Autodesk Inventor part; units mm, degrees
ref_plane "YZ Plane" through (0, 0, 0) normal (1, 0, 0) x (0, 1, 0)
ref_plane "XZ Plane" through (0, 0, 0) normal (0, 1, 0) x (-1, 0, 0)
ref_plane "XY Plane" through (0, 0, 0) normal (0, 0, 1) x (1, 0, 0)
sketch "Sketch1" plane through (0, 0, 0) normal (1, 0, 0) x (0, 1, 0)
  line L0 (0, 0) -> (57.15, 0)
  line L1 (57.15, 0) -> (57.15, 27.94)
  line L2 (0, 0) -> (0, 27.94)
  arc A0 (8.89, 27.94) -> (48.26, 27.94) centre (28.575, 49.4224) ccw
  line L3 (28.575, 0) -> (28.575, 8.5438) construction
  circle A1 centre (3.81, 3.81) radius 1.4
  circle A2 centre (53.34, 3.81) radius 1.4
  line L4 (0, 27.94) -> (5.08, 27.94)
  line L5 (5.08, 27.94) -> (5.08, 26.67)
  line L6 (5.08, 26.67) -> (7.62, 26.67)
  line L7 (7.62, 26.67) -> (7.62, 27.94)
  line L8 (7.62, 27.94) -> (8.89, 27.94)
  line L9 (57.15, 27.94) -> (52.07, 27.94)
  line L10 (52.07, 27.94) -> (52.07, 26.67)
  line L11 (52.07, 26.67) -> (49.53, 26.67)
  line L12 (49.53, 26.67) -> (49.53, 27.94)
  line L13 (49.53, 27.94) -> (48.26, 27.94)
  circle A3 centre (53.34, 24.13) radius 1.4
  circle A4 centre (3.81, 24.13) radius 1.4
  dimension "d0" = 57.15
  dimension "d1" = 27.94
  dimension "d2" = 27.94
  dimension "d3" = 85
  dimension "d4" = 29.1375
  dimension "d5" = 2.8
  dimension "d6" = 3.81
  dimension "d7" = 3.81
  dimension "d8" = 5.08
  dimension "d9" = 1.27
  dimension "d10" = 2.54
  dimension "d11" = 1.27
  dimension "d14" = 2.8
  dimension "d15" = 20.32
  dimension "d16" = 49.4224
  dimension "d17" = 8.89
  dimension "d18" = 49.53
extrude "Extrusion1" add sketch "Sketch1" along normal blind 1
properties part number "PCBModuleLeft01" material "PCB(1)"
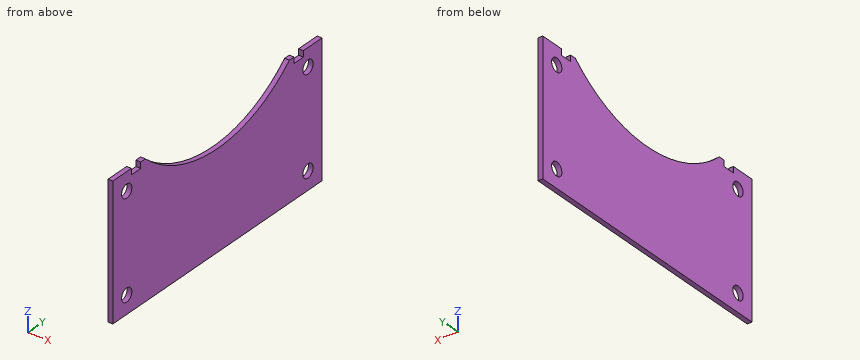
Check sheet for the modelled part. Datum: model origin and axes. Units: mm. Give positions to 0.01 mm unless a question says otherwise; leave off trailing zeros. Loops run counter-clockwise (first coordinate to the right, second up) from the corner with the lowest first, then second, coordinate; pieces in that order, holes last. Notation, with made-up numbers: M 3,-14.75 L 18,-14.75 A22 ccw 18,12.25 Z; hole C 30,39.25 d4. An arc over 180 degrees is marked long. Use a Markdown table: item, result. Add a question column.
Q1. Sectioned sample at A-A, the plane z = 3.81. Record the cut outline in (x, y).
Q2. Scan lines: line 1 along Z through (x, y) = (0.55, 53.34); line 2 along Z through (x, y) = (0.75, 28.5); line 3 along Z through (x, y) = (0.1, 48). Record each from-to range of solid material in increasing order. Write a range as [from, to].
Q3. Sectioned sample at C-C, the plane y = 3.81. Record the cut outline in (x, z), then the cut area to 3 significant figures.
Q4. Sectioned sample at B-B, the plane x = 0.25. Record the cut outline in (y, z) (3 decimals).
Q5. Sectioned sample at D-D, the plane z = 24.13. Record the cut outline in (x, y), then the cut area to 3 significant figures.
Q6. Go/stop test with a flat-tipped pin: pin 1 (1.5 mm diameter, centred on y = 27.5, z = 22, fed in from +X). Record where the tip stops, or that it passes through.
Verdict:
| question | item | result |
|---|---|---|
| 1 | outline | M 0,0 L 1,0 L 1,2.41 L 0,2.41 Z; M 0,5.21 L 1,5.21 L 1,51.94 L 0,51.94 Z; M 0,54.74 L 1,54.74 L 1,57.15 L 0,57.15 Z |
| 2 | line 1 | [0, 2.41], [5.21, 22.73], [25.53, 27.94] |
| 2 | line 2 | [0, 20.29] |
| 2 | line 3 | [0, 27.7] |
| 3 | outline | M 0,0 L 1,0 L 1,2.41 L 0,2.41 Z; M 0,5.21 L 1,5.21 L 1,22.73 L 0,22.73 Z; M 0,25.53 L 1,25.53 L 1,27.94 L 0,27.94 Z |
| 3 | area | 22.3 mm^2 |
| 4 | outline | M 0,0 L 57.15,0 L 57.15,27.94 L 52.07,27.94 L 52.07,26.67 L 49.53,26.67 L 49.53,27.94 L 48.26,27.94 A29.137 cw 8.89,27.94 L 7.62,27.94 L 7.62,26.67 L 5.08,26.67 L 5.08,27.94 L 0,27.94 Z; hole C 3.81,3.81 d2.8; hole C 3.81,24.13 d2.8; hole C 53.34,3.81 d2.8; hole C 53.34,24.13 d2.8 |
| 5 | outline | M 0,0 L 1,0 L 1,2.41 L 0,2.41 Z; M 0,5.21 L 1,5.21 L 1,14.11 L 0,14.11 Z; M 0,43.04 L 1,43.04 L 1,51.94 L 0,51.94 Z; M 0,54.74 L 1,54.74 L 1,57.15 L 0,57.15 Z |
| 5 | area | 22.6 mm^2 |
| 6 | pin 1 | through |
